```python
from build123d import *

# Parameters (mm, degrees)
SKETCH1_R           = 4.1
SKETCH1_R_2         = 2.1
BOSS_EXTRUDE1_DEPTH = 2.2
SKETCH2_R           = 5.25
BOSS_EXTRUDE2_DEPTH = 1
SKETCH3_R           = 5.25
SKETCH3_R_2         = 3.1
BOSS_EXTRUDE3_DEPTH = 5
CHAMFER1_SIZE       = 1.15


with BuildPart() as part:
    # Sketch1 → Boss-Extrude1 (new body)
    with BuildSketch(Plane(origin=(0, 0, 0), x_dir=(1, 0, 0), z_dir=(0, 1, 0))):
        with Locations(Location((0, 0, 0), (0, 0, 270))):
            Circle(SKETCH1_R)
        with Locations(Location((0, 0, 0), (0, 0, 270))):
            Circle(SKETCH1_R_2, mode=Mode.SUBTRACT)
    extrude(amount=BOSS_EXTRUDE1_DEPTH)

    # Sketch2 → Boss-Extrude2 (add)
    with BuildSketch(Plane(origin=(0, 2.2, 0), x_dir=(1, 0, 0), z_dir=(0, 1, 0))):
        with Locations(Location((0, 0, 0), (0, 0, 270))):
            Circle(SKETCH2_R)
    extrude(amount=BOSS_EXTRUDE2_DEPTH)

    # Sketch3 → Boss-Extrude3 (add)
    with BuildSketch(Plane(origin=(0, 3.2, 0), x_dir=(1, 0, 0), z_dir=(0, 1, 0))):
        with Locations(Location((0, 0, 0), (0, 0, 270))):
            Circle(SKETCH3_R)
        with Locations(Location((0, 0, 0), (0, 0, 270))):
            Circle(SKETCH3_R_2, mode=Mode.SUBTRACT)
    extrude(amount=BOSS_EXTRUDE3_DEPTH)

    # Chamfer1
    chamfer1_edges = [part.edges().sort_by_distance(p)[0] for p in [
        (0, 2.2, -4.1),
    ]]
    chamfer(chamfer1_edges, length=CHAMFER1_SIZE - 0.0001)  # a hair under: the kernel refuses the full size


solid = part.part
```
Geometry: final body of the model. Coordinates: model frame, mm. A direction names the side the tool comes from. Coordinates: 2 decimals unless noted, no trailing zeros. Write each loop counter-clockwise with the first axis right and the second up, starting at its lowest first coordinate (ties: lowest second). Pieces come first, ordered by that corner, then holes. Notation, with made-up numbers: M 76.25,8.5 L 109.25,8.5 A26 ccw 109.25,24.5 Z; hole C 9.25,89.5 d2. An arc over 180 degrees is marked long. Answer as CSV lines item,"result". Start each with the question number.
Q1. Reachability of faces 4 (the cylindrical face through (0.931, 5.665, 2.957)), 5 (the flat face through (0, 2.2, 0)), 6 (the flat face through (-2, 0, 2)) from +Z, -Z, +X, -X, +Y, -Y: full face, straight path, thin tool, end or side. Return the list, or none.
Q2. Cut plane C-C on y = 7.25. Return the cut outline in (x, z).
Q3. Pin query (flat end, axial travel): P1, Ø1.3, axis at x = 0.5, z = -0.5, coming from the -Y side; P2, Ø3, axis at x = -1, z = 0, coming from the +Y side; P3, Ø4, axis at x = 2.5, y = 2.5, coming from the +Z side. Return the tip coordinate at first contact, or that it passes through.
Q4. Mould query, pull axis Z, two halves, no side actions, for faces 1 (the cylindrical face through (4.065, 0.518, -0.534)), 2 (the flat face through (-2.3, 8.2, 2.3)), 3 (the cylindrical face through (0.631, 1.085, 2.003)). Classes: released by +Z, released by -Z, zero draft, split by the parting line, or undercut.
Q5. Line query: line 1 (X direction, y = 0.8, z = 0); line 2 (X direction, y = 3.5, z = 0); line 3 (Z direction, x = 0.5, y = 3.25). Output: solid intervals per line, ascending. Write a range as from..to.
Q6. Cut plane D-D on y = 1.5. Return the cut outline in (x, z), then the cut area to 3 significant figures.
Findings below:
1,face 4,"+Y"
1,face 5,"-Y"
1,face 6,"+Z, -Z, +X, -X, -Y"
2,outline,"C 0,0 d10.5; hole C 0,0 d6.2"
3,P1,"stops at y = 2.2"
3,P2,"stops at y = 3.2"
3,P3,"stops at z = 5.23"
4,face 1,"split by the parting line"
4,face 2,"zero draft"
4,face 3,"undercut"
5,line 1,"x = -4.1..-2.1, 2.1..4.1"
5,line 2,"x = -5.25..-3.1, 3.1..5.25"
5,line 3,"z = -5.23..-3.06, 3.06..5.23"
6,outline,"C 0,0 d9.1; hole C 0,0 d4.2"
6,area,"51.2 mm2"
